Input: part model. Units: mm. Frame: model coordinates. A direction names the side the tool comes from. Round coordinates to 2 decimals unless told otherwise and drop trailing zeros. Loops run counter-clockwise (first coordinate to the right, second up) from the corner with the lowest first, then second, coordinate; pieces in that order, holes last. Notation, with made-up numbers: M 29.25,10 L 44.25,10 A29 cw 44.25,40 Z; hole C 60.25,-2 d1. An arc over 180 degrees is marked long. Return JSON: item names as keys, results as strings. Group by question number.
1) Mould query, pull axis X, two halves, no side actions, for faces 1 (the face through (38, 0, 12)), 2 (the face through (11, -33, 11.2)), 3 (the face through (-1, 34, 12)). Classes: +X half, -X half, draft (parallel to the pull), parting line (faces both ways), or undercut.
2) Section D-D (y = -8). Output: boundary loops of the cut face in (x, z).
3) Section A-A (x = -23). Output: boundary loops of the cut face in (y, z), plus the area to 3 significant figures.
4) Section C-C (z = 15). Output: boundary loops of the cut face in (x, y).
5) Material intervals for line 1 (Z direction, x = -17.1, y = -33.45); line 2 (Y direction, x = 12.5, z = 7); line 3 (X direction, y = 19, z = 9.75), sorted ascending. Write a range as from..to.
6) Access query for faces 4 (the face through (28, 33, 8)), 5 (the face through (-1, 32, 13)), 6 (the face through (15, -33, 14)). Directions: +Z, -Z, +X, -X, +Y, -Y. A direction counts if a zero-diameter tool reaches every point of the face in a straight line with its end or side. Return the directions, or none.
7) Section B-B (x = 12). Output: boundary loops of the cut face in (y, z).
8) Contact query for flat-ended pins moving along their axis: P1, Ø6, axis at x = 0.5, y = -20.5, coming from the +Z side; P2, Ø6.5, axis at x = -17.1, z = 10.4, coming from the +Y side. Output: stop coordinate, or through.
from build123d import *

# Parameters (mm, degrees)
SKETCH_W        = 76
SKETCH_H        = 68
PAD_DEPTH       = 25
SKETCH001_W     = 72
SKETCH001_H     = 64
POCKET_DEPTH    = 23
SKETCH002_R     = 2.5
SKETCH002_W     = 8
SKETCH002_H     = 5
POCKET001_DEPTH = 2
SKETCH003_W     = 32
SKETCH003_H     = 13
SKETCH003_W_2   = 12
SKETCH003_H_2   = 11
POCKET002_DEPTH = 2


with BuildPart() as part:
    # Sketch → Pad (new body)
    with BuildSketch(Plane.XY):
        Rectangle(SKETCH_W, SKETCH_H)
    extrude(amount=PAD_DEPTH)

    # Sketch001 → Pocket (cut)
    with BuildSketch(Plane.XY.offset(2)):
        Rectangle(SKETCH001_W, SKETCH001_H)
    extrude(amount=POCKET_DEPTH, mode=Mode.SUBTRACT)

    # Sketch002 → Pocket001 (cut)
    with BuildSketch(Plane.XZ.offset(34)):
        with Locations((-7.4, 10.4)):
            Circle(SKETCH002_R)
        with Locations((-17.1, 10.4)):
            Circle(SKETCH002_R)
        with Locations((-26.8, 10.4)):
            Circle(SKETCH002_R)
        with Locations((11, 13.7)):
            Rectangle(SKETCH002_W, SKETCH002_H)
    extrude(amount=-POCKET001_DEPTH, mode=Mode.SUBTRACT)

    # Sketch003 → Pocket002 (cut)
    with BuildSketch(Plane.XZ.offset(-34)):
        with Locations((-20, 12.5)):
            Rectangle(SKETCH003_W, SKETCH003_H)
        with Locations((12, 13.5)):
            Rectangle(SKETCH003_W_2, SKETCH003_H_2)
        with Locations((28, 13.5)):
            Rectangle(SKETCH003_W_2, SKETCH003_H_2)
    extrude(amount=POCKET002_DEPTH, mode=Mode.SUBTRACT)


solid = part.part
Returned:
{
 "1": {"face 1": "+X half", "face 2": "undercut", "face 3": "draft"},
 "2": {"outline": "M -38,0 L 38,0 L 38,25 L 36,25 L 36,2 L -36,2 L -36,25 L -38,25 Z"},
 "3": {"outline": "M -34,0 L 34,0 L 34,6 L 32,6 L 32,2 L -32,2 L -32,25 L -34,25 Z; M 32,19 L 34,19 L 34,25 L 32,25 Z", "area": "202 mm^2"},
 "4": {"outline": "M -38,-34 L 7,-34 L 7,-32 L -36,-32 L -36,34 L -38,34 Z; M -4,32 L 6,32 L 6,34 L -4,34 Z; M 15,-34 L 38,-34 L 38,34 L 34,34 L 34,32 L 36,32 L 36,-32 L 15,-32 Z; M 18,32 L 22,32 L 22,34 L 18,34 Z"},
 "5": {"line 1": "z = 0..7.9, 12.9..25", "line 2": "y = -34..-32, 32..34", "line 3": "x = -38..-36, 36..38"},
 "6": {"face 4": "+Y", "face 5": "+Z", "face 6": "+Y, -Y"},
 "7": {"outline": "M -34,0 L 34,0 L 34,8 L 32,8 L 32,2 L -32,2 L -32,11.2 L -34,11.2 Z; M -34,16.2 L -32,16.2 L -32,25 L -34,25 Z; M 32,19 L 34,19 L 34,25 L 32,25 Z"},
 "8": {"P1": "stops at z = 2", "P2": "stops at y = -32"}
}
